The model under review builds one solid part; all positions refer to its coordinate system, in mm. Coordinates: 2 decimals unless noted, no trailing zeros. Write each loop counter-clockwise with the first axis right and the second up, starting at its lowest first coordinate (ties: lowest second). Pieces come first, ordered by that corner, then holes. Notation, with made-up numbers: (-29.5, 63) -> (-5.5, 63) arc R16 cw to (-5.5, 93) -> close; hole circle Ø2 at (-27, -21.5). An arc over 180 degrees is marked (long way). Write each question's results on one line, items separated by ' | '.
Autodesk Inventor part; units mm, degrees
ref_plane "Work Plane1" through (-101.6, 0, 0) normal (1, 0, 0) x (0, 0, -1)
ref_plane "YZ Plane" through (0, 0, 0) normal (1, 0, 0) x (0, 1, 0)
ref_plane "XZ Plane" through (0, 0, 0) normal (0, 1, 0) x (-1, 0, 0)
sketch "Sketch1" plane through (0, 0, 0) normal (0, 0, 1) x (1, 0, 0)
  line L0 (0, 0) -> (-203.2, 0)
  line L1 (-203.2, 0) -> (-203.2, 127)
  line L2 (-203.2, 127) -> (0, 127)
  line L3 (0, 127) -> (0, 0)
  dimension "d0" = 127
  dimension "d1" = 203.2
extrude "Extrusion1" add sketch "Sketch1" along normal blind 3.175
sketch "Sketch2" plane through (0, 0, 3.175) normal (0, 0, 1) x (1, 0, 0)
  circle A0 centre (-69.85, 50.8) radius 14.2875
  line L0 (0, 0) -> (0, 127)
  line L1 (-203.2, 0) -> (0, 0)
  circle A1 centre (-133.35, 50.8) radius 14.2875
  line L2 (-101.6, 0) -> (-101.6, 50.8)
  line L3 (-101.6, 50.8) -> (-69.85, 50.8)
  line L4 (-69.85, 50.8) -> (-133.35, 50.8)
  dimension "d4" = 28.575
  dimension "d8" = 28.575
  dimension "d9" = 50.8
  dimension "d28" = 63.5
  dimension "d29" = 31.75
extrude "Extrusion2" cut sketch "Sketch2" against normal blind 3.175
sketch "Sketch3" plane through (0, 0, 3.175) normal (0, 0, 1) x (1, 0, 0)
  circle A0 centre (-6.35, 6.35) radius 3.175
  line L0 (0, 0) -> (0, 127)
  line L1 (-203.2, 0) -> (0, 0)
  circle A1 centre (-6.35, 120.65) radius 3.175
  line L2 (0, 127) -> (-203.2, 127)
  circle A2 centre (-196.85, 120.65) radius 3.175
  circle A3 centre (-196.85, 6.35) radius 3.175
  line L3 (-203.2, 127) -> (-203.2, 0)
  dimension "d12" = 6.35
  dimension "d13" = 6.35
  dimension "d14" = 6.35
  dimension "d15" = 6.35
  dimension "d16" = 6.35
  dimension "d17" = 6.35
  dimension "d18" = 6.35
  dimension "d19" = 6.35
  dimension "d20" = 6.35
  dimension "d30" = 6.35
  dimension "d31" = 6.35
  dimension "d32" = 6.35
hole "Hole1" at (-196.85, 120.65, 3.175) at (-196.85, 6.35, 3.175) at (-6.35, 6.35, 3.175) at (-6.35, 120.65, 3.175) direction (0, 0, -1) diameter 6.35 end through all
ref_plane "Work Plane1" through (-101.6, 0, 0) normal (1, 0, 0) x (0, 0, -1)
sketch "Sketch4" plane through (0, 0, 3.175) normal (0, 0, 1) x (1, 0, 0)
  circle A0 centre (-69.85, 50.8) radius 14.2875
  line L0 (-69.85, 50.8) -> (-41.0234, 79.6266)
  line L1 (-69.85, 50.8) -> (-23.1148, 50.8)
  circle A1 centre (-41.0234, 79.6266) radius 12.7
  point P0 (0, 0)
  dimension "d33" = 40.767
  dimension "d34" = 315
  dimension "d35" = 25.4
extrude "Extrusion3" cut sketch "Sketch4" against normal through all contours A1
sketch "Sketch5" plane through (0, 0, 3.175) normal (0, 0, 1) x (1, 0, 0)
  circle A0 centre (-41.0234, 79.6266) radius 12.7
  line L0 (-41.0234, 79.6266) -> (-27.001, 58.448)
  line L1 (-41.0234, 79.6266) -> (-19.8448, 93.649)
  line L2 (-41.0234, 79.6266) -> (-55.0458, 100.8052)
  circle A1 centre (-55.0458, 100.8052) radius 1.9844
  circle A2 centre (-19.8448, 93.649) radius 1.9844
  circle A3 centre (-27.001, 58.448) radius 1.9844
  point P0 (0, 0)
  dimension "d38" = 25.4
  dimension "d39" = 25.4
  dimension "d40" = 25.4
  dimension "d41" = 3.9688
  dimension "d42" = 3.9688
  dimension "d43" = 3.9688
extrude "Extrusion4" cut sketch "Sketch5" against normal blind 25.4 contours A3 | A1
equation "\"d29\" = 0.5 * d28"
properties part number "Gearbox plate"
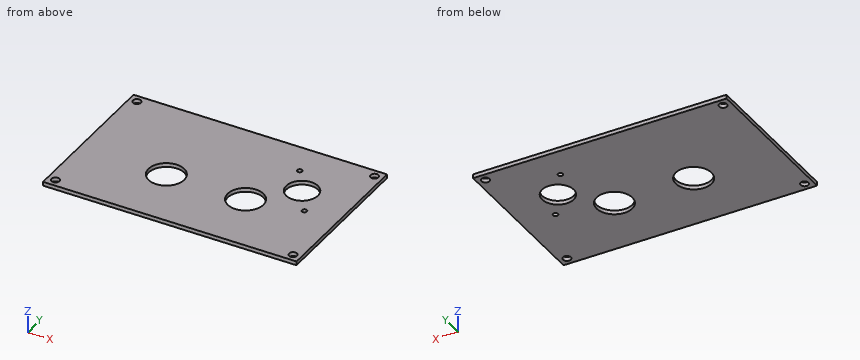
Q1. Clearance check with flat-ended pins moving along their axes: P1, Ø1.5, axis at x = -150.5, z = 2, coming from the -Y side; P2, Ø5, axis at x = -6.35, y = 6.35, coming from the -Z side. State where each tip first meets the part, or that it passes through.
Solution:
P1: y = 0 | P2: through
Q2. For line 1 (Y direction, x = -6.35, z = 1.95) (3 decimals); line 2 (X direction, y = 120.65, z = 1.5) (3 decimals); line 3 (Y direction, x = -133.35, z = 2), list the stretches that pass through material, from the lowest coordinate up. Write a range as from..to.
Solution:
line 1: 0..3.175, 9.525..117.475, 123.825..127 | line 2: -203.2..-200.025, -193.675..-9.525, -3.175..0 | line 3: 0..36.51, 65.09..127
Q3. Add section B-B (x = -133.35). Write out the cut boundary in (y, z) (1 decimal), plus the area to 4 significant figures.
Solution:
outline: (0, 0) -> (36.5, 0) -> (36.5, 3.2) -> (0, 3.2) -> close; (65.1, 0) -> (127, 0) -> (127, 3.2) -> (65.1, 3.2) -> close | area: 312.5 mm²
Q4. Add section D-D (z = 0.95). Count the separate pieces of the cut face and the enclosed holes in it, plus the area to 3 significant figures.
Solution:
separate pieces: 1 | enclosed holes: 9 | area: 23,900 mm²
Q5. Add section A-A (x = -196.85). Write out the cut boundary in (y, z) (3 decimals).
Solution:
outline: (0, 0) -> (3.175, 0) -> (3.175, 3.175) -> (0, 3.175) -> close; (9.525, 0) -> (117.475, 0) -> (117.475, 3.175) -> (9.525, 3.175) -> close; (123.825, 0) -> (127, 0) -> (127, 3.175) -> (123.825, 3.175) -> close
Q6. Add section C-C (y = 88). Write out the cut boundary in (x, z) (3 decimals), plus the area to 3 significant figures.
Solution:
outline: (-203.2, 0) -> (-50.572, 0) -> (-50.572, 3.175) -> (-203.2, 3.175) -> close; (-31.475, 0) -> (0, 0) -> (0, 3.175) -> (-31.475, 3.175) -> close | area: 585 mm²
